```python
from build123d import *

# Parameters (mm, degrees)
ESQUISSE1_R        = 2.5
BOSS_EXTRU_1_DEPTH = 10
ESQUISSE1_3_R      = 2.5
BOSS_EXTRU_2_DEPTH = 13
CONG_1_R           = 1
ESQUISSE1_4_W      = 3
ESQUISSE1_4_H      = 25
BOSS_EXTRU_3_DEPTH = 2


with BuildPart() as part:
    # Esquisse1 → Boss.-Extru.1 (new body)
    # profile 1 of 4: a face of its own
    with BuildSketch(Plane.XY):
        Polygon((-32.758882294, 65.250907441), (-32.758882294, 62.500907441), (101.241117706, 62.500907441), (101.241117706, 72.500907441), (-32.758882294, 72.500907441), (-32.758882294, 69.750907441), (-27.258882294, 69.750907441), (-27.258882294, 65.250907441), align=None)
        with Locations((31.241117706, 67.500907441)):
            Circle(ESQUISSE1_R, mode=Mode.SUBTRACT)
    # profile 2 of 4: a face of its own
    with BuildSketch(Plane.XY):
        with BuildLine():
            ThreePointArc((101.241117706, 72.500907441), (121.410045947, -12.499092559), (101.241117706, -97.499092559))
            Line((101.241117706, -97.499092559), (101.241117706, -87.499092559))
            ThreePointArc((101.241117706, -87.499092559), (111.410045947, -12.499092559), (101.241117706, 62.500907441))
            Line((101.241117706, 62.500907441), (101.241117706, 72.500907441))
        make_face()
        with Locations((116.410045947, -12.499092559)):
            Circle(ESQUISSE1_R, mode=Mode.SUBTRACT)
    # profile 3 of 4: a face of its own
    with BuildSketch(Plane.XY):
        Polygon((-32.758882294, -97.499092559), (101.241117706, -97.499092559), (101.241117706, -87.499092559), (-32.758882294, -87.499092559), (-32.758882294, -90.249092559), (-27.258882294, -90.249092559), (-27.258882294, -94.749092559), (-32.758882294, -94.749092559), align=None)
        with Locations((31.241117706, -92.499092559)):
            Circle(ESQUISSE1_R, mode=Mode.SUBTRACT)
    # profile 4 of 4: a face of its own
    with BuildSketch(Plane.XY):
        with BuildLine():
            Line((111.910045947, 0.000907441), (111.132538059, 0.000907441))
            ThreePointArc((111.132538059, 0.000907441), (111.410045947, -12.499092559), (111.132538059, -24.999092559))
            Line((111.132538059, -24.999092559), (111.910045947, -24.999092559))
            Line((111.910045947, -24.999092559), (111.910045947, 0.000907441))
        make_face()
    extrude(amount=BOSS_EXTRU_1_DEPTH)

    # Esquisse1_3 → Boss.-Extru.2 (add)
    with BuildSketch(Plane.XY):
        with Locations(Location((31.241117706, 67.500907441, 0), (0, 0, 180))):
            Circle(ESQUISSE1_3_R)
        with Locations(Location((116.410045947, -12.499092559, 0), (0, 0, 180))):
            Circle(ESQUISSE1_3_R)
        with Locations(Location((31.241117706, -92.499092559, 0), (0, 0, 180))):
            Circle(ESQUISSE1_3_R)
    extrude(amount=BOSS_EXTRU_2_DEPTH)

    # Cong_1
    cong_1_edges = [part.edges().sort_by_distance(p)[0] for p in [
        (33.741117706, 67.500907441, 13),
        (118.910045947, -12.499092559, 13),
        (33.741117706, -92.499092559, 13),
    ]]
    fillet(cong_1_edges, radius=CONG_1_R)

    # Esquisse1_4 → Boss.-Extru.3 (add)
    with BuildSketch(Plane.XY):
        with Locations((110.410045947, -12.499092559)):
            Rectangle(ESQUISSE1_4_W, ESQUISSE1_4_H)
    extrude(amount=BOSS_EXTRU_3_DEPTH)


solid = part.part
```
Design review of the part built by this model. Coordinates are the model's own, in mm. A direction names the side the tool comes from. Round coordinates to 2 decimals unless told otherwise and drop trailing zeros. Order: outer loops, then holes, each group sorted by start corner. A loop starts at its lowest first (then second) coordinate and runs counter-clockwise, first axis right, second up. Notation, with made-up numbers: M 32,9.25 L 80,9.25 A24 ccw 80,26.25 Z; hole C 73,1 d4. An arc over 180 degrees is marked long. Put each result on its own line as item: value.
Q1. Consider section C-C (y = 12). State the section outline as (x, z) points.
Reported:
outline: M 110.34,0 L 119.82,0 L 119.82,10 L 110.34,10 Z
Q2. Draft analysis for pull direction Y (two halves, no side actions). For faces 4 (the face through (35, 72.501, 5)), 5 (the face through (35, -87.499, 5)), 6 (the face through (118.908, -12.609, 10.986)), 7 (the face through (-27.259, 68, 5)), state which applies: released by +Y, released by -Y, zero draft, split by the parting line, or undercut.
Reported:
face 4: released by +Y
face 5: undercut
face 6: split by the parting line
face 7: undercut
Q3. Consider section D-D (y = -51.5). State the section outline as (x, z) points, and give its area (3 significant figures).
Reported:
outline: M 108.7,0 L 117.35,0 L 117.35,10 L 108.7,10 Z
area: 86.5 mm²
Q4. Consider section A-A (x = -10). State the section outline as (y, z) points, and give its area (3 significant figures).
Reported:
outline: M -97.5,0 L -87.5,0 L -87.5,10 L -97.5,10 Z; M 62.5,0 L 72.5,0 L 72.5,10 L 62.5,10 Z
area: 200 mm²
Q5. Machinability: for faces 1 (the face through (-30, -90.249, 5)), 2 (the face through (33, -97.499, 5)), 3 (the face through (28.857, 66.75, 10.986)), which of the approach directions +Z, -Z, +X, -X, +Y, -Y give a long, thin tool a straight path to every point of the face, cutting with its end or side? Answer none if there is none.
Reported:
face 1: +Z, -Z, -X
face 2: +Z, -Z, +X, -X, -Y
face 3: +Z
Q6. Insertion check: pin 1 Ø1.2 at (x, y) = (110.5, -17.5) entering from +Z; pin 2 Ø2 at (y, z) = (68, 4) entering from -X; pin 3 Ø1 at (y, z) = (-11, 1.5) entering from -X. Each pin has a flat end and moves straight along its axis. Give the tip position at first contact, or say it passes through.
Reported:
pin 1: z = 2
pin 2: x = -27.26
pin 3: x = 108.91
Q7. Consider section B-B (z = 5.5). State the section outline as (x, y) points.
Reported:
outline: M -32.76,-97.5 L 101.24,-97.5 A189.2 ccw 101.24,72.5 L -32.76,72.5 L -32.76,69.75 L -27.26,69.75 L -27.26,65.25 L -32.76,65.25 L -32.76,62.5 L 101.24,62.5 A281.66 cw 101.24,-87.5 L -32.76,-87.5 L -32.76,-90.25 L -27.26,-90.25 L -27.26,-94.75 L -32.76,-94.75 Z
Q8. To check wall thickness, follow line 1 (Y direction, x = 84, z = 5.25); line 2 (X direction, y = -9, z = 9.25); line 3 (Y direction, x = 30, z = 11.25). State the ranges of each line that lie inside material, in increasing order.
Reported:
line 1: -97.5 to -87.5, 62.5 to 72.5
line 2: 111.39 to 121.38
line 3: -94.67 to -90.33, 65.33 to 69.67
